Design review of the part shown in the three views and the two pictorial views. Dimensions are in mm from the part's minimum x, y and z. A direction names the side the tool comes from. Round coordinates to 2 decimals unless told otherwise and drop trailing zeros. Write each loop counter-clockwise with the first axis right and the second up, starting at its lowest first coordinate (ties: lowest second). Pieces come first, ordered by that corner, then holes. Notation, with made-up numbers: (64, -25) -> (76, -25) arc R31 cw to (76, 2) -> close; hole circle Ø7 at (-29, 62). An arc over 180 degrees is marked (long way). Answer as a JSON object with one key per item and string values. Group by question number.
1) Insertion check: pin 1 Ø11.5 at (x, y) = (36.5, 21) entering from +Z; pin 2 Ø10 at (x, z) = (17.5, 31) entering from -Y; pin 3 Ø4 at (y, z) = (12.5, 3.5) entering from +X; pin 4 Ø2 at (x, y) = (50, 23.5) entering from +Z. Each pin has a flat end and moves straight along its axis. Give the tip position at first contact, or say it passes through.
2) We need section C-C, the plane y = 21. Write out the cut boundary in (x, z).
3) To check wall thickness, follow probe 1 along X at (y, z) = (19, 20); probe 2 along Z at (x, y) = (13, 17); probe 3 along Z at (x, y) = (12, 5.5). State the ranges of each line that lie inside material, in increasing order. Write a range as [from, to].
4) We need section B-B, the plane x = 53.5. Write out the cut boundary in (y, z), then the cut area to 3 significant figures.
5) We need section A-A, the plane z = 24. Write out the cut boundary in (x, y).
6) Machinability: for the marked faces 5, 6 and 7, which of the approach directions +Z, -Z, +X, -X, +Y, -Y give a long, thin tool a straight path to every point of the face, cutting with its end or side? Answer none if there is none.
7) Mouldability with a two-part tool opening along X and no side actions: class the marked faces 1, 2, 3 and 4 as pulls with the +X half, pulls with the -X half, needs draft (parallel to the pull), parting line crosses it, or undercut.
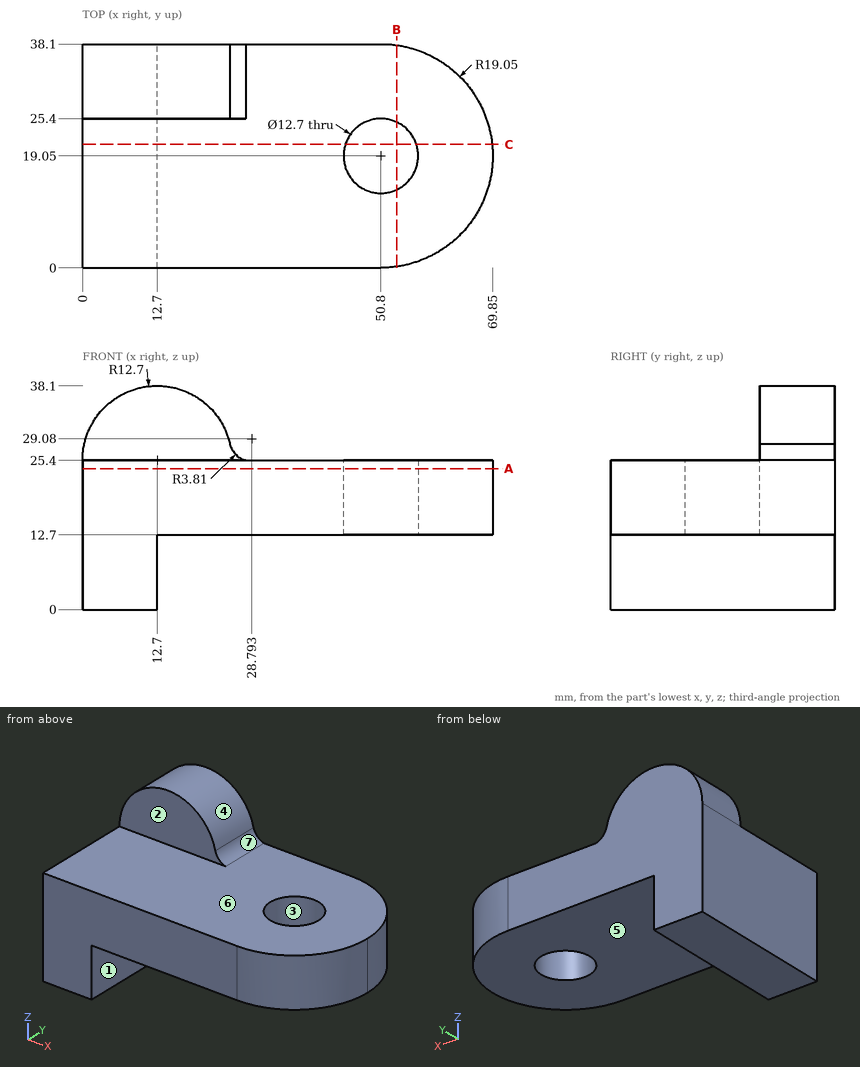
Here are the results:
{
 "1": {"pin 1": "stops at z = 25.4", "pin 2": "stops at y = 25.4", "pin 3": "stops at x = 12.7", "pin 4": "passes through"},
 "2": {"outline": "(0, 0) -> (12.7, 0) -> (12.7, 12.7) -> (44.76, 12.7) -> (44.76, 25.4) -> (0, 25.4) -> close; (56.84, 12.7) -> (69.75, 12.7) -> (69.75, 25.4) -> (56.84, 25.4) -> close"},
 "3": {"probe 1": "x = [0, 44.45], [57.15, 69.85]", "probe 2": "z = [12.7, 25.4]", "probe 3": "z = [0, 25.4]"},
 "4": {"outline": "(0.19, 12.7) -> (13.3, 12.7) -> (13.3, 25.4) -> (0.19, 25.4) -> close; (24.8, 12.7) -> (37.91, 12.7) -> (37.91, 25.4) -> (24.8, 25.4) -> close", "area": "333 mm^2"},
 "5": {"outline": "(0, 0) -> (50.8, 0) arc R19.05 ccw to (69.85, 19.05) arc R19.05 ccw to (50.8, 38.1) -> (0, 38.1) -> close; hole circle Ø12.7 at (50.8, 19.05)"},
 "6": {"face 5": "-Z, +X, +Y, -Y", "face 6": "+Z, +X, -Y", "face 7": "+Z, +X, +Y, -Y"},
 "7": {"face 1": "pulls with the +X half", "face 2": "needs draft", "face 3": "undercut", "face 4": "parting line crosses it"}
}
